from build123d import *

# Parameters (mm, degrees)
BASE_FLANGE1_DEPTH             = 1.15
TAB1_DEPTH                     = 0.35
F_3_2_3_2_DIAMETER_HOLE1_D     = 3.2
F_1_4_1_4_DIAMETER_HOLE1_D     = 1.4
F_1_4_1_4_DIAMETER_HOLE1_DEPTH = 0.35
CUT_EXTRUDE1_DEPTH             = 10


# Sheet-metal steps are written as plain solids
with BuildPart() as part:
    # Sketch80 → Base-Flange1 (new, symmetric)
    with BuildSketch(Plane.XY):
        with BuildLine():
            Line((3.744076121, -16.948565679), (2.751685988, -15.763663573))
            ThreePointArc((2.751685988, -15.763663573), (2.602525969, -15.289062626), (2.832647456, -14.847997018))
            Line((2.832647456, -14.847997018), (3.949719342, -13.912416676))
            ThreePointArc((3.949719342, -13.912416676), (3.974169718, -13.88200963), (3.985122647, -13.844560429))
            Line((3.985122647, -13.844560429), (5.199611389, -0.108807447))
            ThreePointArc((5.199611389, -0.108807447), (5.17375888, -0.032474985), (5.1, 0))
            Line((5.1, 0), (-5.1, 0))
            ThreePointArc((-5.1, 0), (-5.17375888, -0.032474985), (-5.199611389, -0.108807447))
            Line((-5.199611389, -0.108807447), (-3.985122647, -13.844560429))
            ThreePointArc((-3.985122647, -13.844560429), (-3.974169718, -13.88200963), (-3.949719342, -13.912416676))
            Line((-3.949719342, -13.912416676), (-2.832647456, -14.847997018))
            ThreePointArc((-2.832647456, -14.847997018), (-2.602525969, -15.289062626), (-2.751685988, -15.763663573))
            Line((-2.751685988, -15.763663573), (-3.744076121, -16.948565679))
            Line((-3.744076121, -16.948565679), (-4.01239905, -16.723837386))
            Line((-4.01239905, -16.723837386), (-3.020008918, -15.53893528))
            ThreePointArc((-3.020008918, -15.53893528), (-2.951165832, -15.319888689), (-3.057375749, -15.116319947))
            Line((-3.057375749, -15.116319947), (-4.174447634, -14.180739606))
            ThreePointArc((-4.174447634, -14.180739606), (-4.284474328, -14.043907898), (-4.33376251, -13.875386492))
            Line((-4.33376251, -13.875386492), (-5.548251252, -0.13963351))
            ThreePointArc((-5.548251252, -0.13963351), (-5.431914959, 0.203862568), (-5.1, 0.35))
            Line((-5.1, 0.35), (5.1, 0.35))
            ThreePointArc((5.1, 0.35), (5.431914959, 0.203862568), (5.548251252, -0.13963351))
            Line((5.548251252, -0.13963351), (4.33376251, -13.875386492))
            ThreePointArc((4.33376251, -13.875386492), (4.284474328, -14.043907898), (4.174447634, -14.180739606))
            Line((4.174447634, -14.180739606), (3.057375749, -15.116319947))
            ThreePointArc((3.057375749, -15.116319947), (2.951165832, -15.319888689), (3.020008918, -15.53893528))
            Line((3.020008918, -15.53893528), (4.01239905, -16.723837386))
            Line((4.01239905, -16.723837386), (3.744076121, -16.948565679))
        make_face()
    extrude(amount=BASE_FLANGE1_DEPTH, both=True)

    # Sketch81 → Tab1 (add)
    with BuildSketch(Plane(origin=(0, 0.35, 0), x_dir=(1, 0, 0), z_dir=(0, 1, 0))):
        with BuildLine():
            Line((-1.636306817, 1.15), (1.636306817, 1.15))
            ThreePointArc((1.636306817, 1.15), (0, 2), (-1.636306817, 1.15))
        make_face()
        with BuildLine():
            Line((-1.636306817, -1.15), (1.636306817, -1.15))
            ThreePointArc((1.636306817, -1.15), (0, -2), (-1.636306817, -1.15))
        make_face()
    extrude(amount=-TAB1_DEPTH)

    # Ø3.2 (3.2) Diameter Hole1 (through all)
    with Locations(Plane(origin=(0, 0.35, 0), x_dir=(1, 0, 0), z_dir=(0, 1, 0))):
        with Locations((0, 0)):
            Hole(F_3_2_3_2_DIAMETER_HOLE1_D / 2)

    # Ø1.4 (1.4) Diameter Hole1
    with Locations(Plane(origin=(0, 0.35, 0), x_dir=(1, 0, 0), z_dir=(0, 1, 0))):
        with Locations((-3.5, 0), (3.5, 0)):
            Hole(F_1_4_1_4_DIAMETER_HOLE1_D / 2, depth=F_1_4_1_4_DIAMETER_HOLE1_DEPTH)

    # Sketch90 → Cut-Extrude1 (cut)
    with BuildSketch(Plane(origin=(-5.873973903, -4.919624761, 0), x_dir=(0, 0, -1), z_dir=(0.7666369409597348, 0.6420808366209819, 0))):
        with BuildLine():
            Line((-1.15, -15.897396074), (-1.15, -14.247396074))
            ThreePointArc((-1.15, -14.247396074), (0, -15.397396074), (1.15, -14.247396074))
            Line((1.15, -14.247396074), (1.15, -15.897396074))
            Line((1.15, -15.897396074), (-1.15, -15.897396074))
        make_face()
    cut_extrude1 = extrude(amount=-CUT_EXTRUDE1_DEPTH, mode=Mode.SUBTRACT)

    # Mirror1: Cut-Extrude1 across plane
    add(cut_extrude1.mirror(Plane(origin=(0, 0, 0), x_dir=(0, 0, 1), z_dir=(1, 0, 0))), mode=Mode.SUBTRACT)


solid = part.part
Design review of the part built by this model. Coordinates are the model's own, in mm. A direction names the side the tool comes from. Round coordinates to 2 decimals unless told otherwise and drop trailing zeros. Write each loop counter-clockwise with the first axis right and the second up, starting at its lowest first coordinate (ties: lowest second). Pieces come first, ordered by that corner, then holes.
Item 1: Consider section B-B on y = -3.5. Give the boundary of the cut face in (x, z), and give its area (3 significant figures).
Item 2: For pin 1 Ø1 at (y, z) = (-5.5, -1.5) entering from +X; pin 2 Ø2 at (x, y) = (4, -5) entering from -Z; pin 3 Ø1.5 at (y, z) = (-7.5, 0.5) entering from -X, all flat-tipped, find the tip position at first contact; note any pin that passes through.
Item 3: For faces 1 (the flat face through (3.14, -16.23, 0.02)), 2 (the flat face through (-4.9, -5.4, 1.15)), 3 (the flat face through (-4.9, -5.4, -1.15)), 4 (the flat face through (4.8, -6.6, -1.15)), list the 3-axis set-ups (+Z, -Z, +X, -X, +Y, -Y) from which the entire face can be reached by the end or side of a thin tool; tool diameter is ignored.
Item 4: Draft analysis for pull direction Z (two halves, no side actions). For faces 5 (the cylindrical face through (-2.8, 0.17, -0.03)), 6 (the cylindrical face through (0.03, 0.18, -2)), 7 (the flat face through (3.624, -14.642, 0.016)), state which applies: released by +Z, released by -Z, zero draft, split by the parting line, or undercut.
Item 5: Consider section C-C on z = 0. Count the separate pieces of the cut face and the enclosed holes in it, and give its area (3 significant figures).
Item 6: Wall thickness on L1, parallel to Y at x = -1.75, z = -0.9; L2, parallel to Z at x = -3.5, y = 0.2; L3, parallel to X at y = -6.25, z = 0.85: over which ranges is each line inside the solid? List them lowest first.
Item 7: Consider section A-A on x = 0. Give the boundary of the cut face in (y, z), and give its area (3 significant figures).
Item 8: Consider section D-D on x = 2.25. Give the boundary of the cut face in (y, z).
Check values:
1. outline: (-5.25, -1.15) - (-4.9, -1.15) - (-4.9, 1.15) - (-5.25, 1.15) - close; (4.9, -1.15) - (5.25, -1.15) - (5.25, 1.15) - (4.9, 1.15) - close
1. area: 1.62 mm2
2. pin 1: stops at x = 5.11
2. pin 2: stops at z = -1.15
2. pin 3: stops at x = -4.96
3. face 1: +Z, -Z, -Y
3. face 2: +Z, -X, +Y, -Y
3. face 3: -Z, -X, +Y, -Y
3. face 4: -Z, +X, +Y, -Y
4. face 5: undercut
4. face 6: released by -Z
4. face 7: zero draft
5. separate pieces: 4
5. enclosed holes: 0
5. area: 14.2 mm2
6. L1: y = 0 to 0.35
6. L2: z = -1.15 to -0.7, 0.7 to 1.15
6. L3: x = -5.01 to -4.66, 4.66 to 5.01
7. outline: (0, -2) - (0.35, -2) - (0.35, -1.6) - (0, -1.6) - close; (0, 1.6) - (0.35, 1.6) - (0.35, 2) - (0, 2) - close
7. area: 0.280 mm2
8. outline: (0, -1.15) - (0.35, -1.15) - (0.35, 1.15) - (0, 1.15) - close
